```python
from build123d import *

# Parameters (mm, degrees)
F0_R        = 9.525
F1_DEPTH    = 44.45
F2_T1_DEPTH = 44.45
F3_R        = 9.525
F4_W        = 58.7756
F4_H        = 15.875
F5_DEPTH    = 25.4
F6_T1_DEPTH = 12.7


# Not quite as in the source:
# - a fillet or chamfer that OpenCascade refuses, or shapes differently, is made with other operations: its cross-section is extruded or revolved along the edge and cut away or added


with BuildPart() as f1:
    # F0 (on Top) → F1 (new body)
    with BuildSketch(Plane.XY):
        with BuildLine():
            ThreePointArc((0, 19.05), (10.9985226281, 15.5542598667), (17.9605122421, 6.35))
            Line((17.9605122421, 6.35), (88.9, 6.35))
            Line((88.9, 6.35), (88.9, 19.05))
            Line((88.9, 19.05), (0, 19.05))
        make_face()
        with BuildLine():
            ThreePointArc((0, 19.05), (-13.4703841816, -13.4703841816), (19.05, 0))
            ThreePointArc((19.05, 0), (18.7756525614, 3.2213926947), (17.9605122421, 6.35))
            ThreePointArc((17.9605122421, 6.35), (10.9985226281, 15.5542598667), (0, 19.05))
        make_face()
        Circle(F0_R, mode=Mode.SUBTRACT)
    extrude(amount=F1_DEPTH)

    # F2: fillet of radius 6.35 on 1 edges, made by hand

    # F2_s2 → F2_t1 (join)
    with BuildSketch(Plane.XY):
        with BuildLine():
            ThreePointArc((25.4, 6.35), (20.9098719395, 4.4901280605), (19.05, 0))
            ThreePointArc((19.05, 0), (18.7756525614, 3.2213926947), (17.9605122421, 6.35))
            Line((17.9605122421, 6.35), (25.4, 6.35))
        make_face()
    extrude(amount=F2_T1_DEPTH)

    # F3
    f3_edges = [f1.edges().sort_by_distance(p)[0] for p in [
        (88.9, 12.7, 44.45),
        (88.9, 12.7, 0),
    ]]
    fillet(f3_edges, radius=F3_R)

    # F4 (on face) → F5 (cut)
    with BuildSketch(Plane.XZ.offset(-6.35)):
        with Locations((59.5122, 22.2023769543)):
            Rectangle(F4_W, F4_H)
    extrude(amount=-F5_DEPTH, mode=Mode.SUBTRACT)

    # F6: fillet of radius 7.9756 on 2 edges, made by hand

    # F6_s2 → F6_t1 (join)
    with BuildSketch(Plane.XZ.offset(-19.05)):
        with BuildLine():
            ThreePointArc((30.1244, 22.1642769543), (32.460399156, 27.8038777983), (38.1, 30.1398769543))
            Line((38.1, 30.1398769543), (30.1244, 30.1398769543))
            Line((30.1244, 30.1398769543), (30.1244, 22.1642769543))
        make_face()
        with BuildLine():
            ThreePointArc((38.1, 14.2648769543), (32.460399156, 16.6008761102), (30.1244, 22.2404769543))
            Line((30.1244, 22.2404769543), (30.1244, 14.2648769543))
            Line((30.1244, 14.2648769543), (38.1, 14.2648769543))
        make_face()
    extrude(amount=F6_T1_DEPTH)


solid = f1.part
```
For this review, take the finished solid that the model builds, in its own axes (mm). A direction names the side the tool comes from. Coordinates: 2 decimals unless noted, no trailing zeros. Loops run counter-clockwise (first coordinate to the right, second up) from the corner with the lowest first, then second, coordinate; pieces in that order, holes last. Notation, with made-up numbers: (85, 19.25) -> (119, 19.25) arc R17 cw to (119, 29.25) -> close; hole circle Ø11 at (79.5, 66.5). An arc over 180 degrees is marked (long way). Return JSON: item names as keys, results as strings. Group by question number.
(1) Consider section C-C, the plane z = 11.5. Give the boundary of the cut face in (x, y) (3 decimals).
(2) Tool access review of faces 4 (the flat face through (44, 19.05, 32)), 5 (the flat face through (63, 13, 14.265)): name each direction out of +Z, -Z, +X, -X, +Y, -Y from which nothing blocks a thin tool from reaching the whole face with its end or side.
(3) Consider section A-A, the plane x = 56. Give the boundary of the cut face in (y, z).
(4) Consider section B-B, the plane y = -6. Give the boundary of the cut face in (x, z).
(5) For pin 1 Ø1 at (x, z) = (52.5, 14) entering from -Y; pin 2 Ø3 at (y, z) = (-10.5, 32) entering from +X, all flat-tipped, find the tip position at first contact; note any pin that passes through.
(6) To check wall thickness, follow L1, parallel to Y at x = 0, z = 22 (3 decimals); L2, parallel to Z at x = 70, y = 14; L3, parallel to X at y = -0.5, z = 11. State the ranges of each line that lie inside material, in increasing order.
(7) Mouldability with a two-part tool opening along Y and no side actions: class faces 1 (the cylindrical face through (-7.559, -5.796, 21.914)), 2 (the cylindrical face through (32.412, 12.789, 27.755)), 3 (the flat face through (57, 6.35, 32)) as pulls with the +Y half, pulls with the -Y half, needs draft (parallel to the pull), parting line crosses it, or undercut.
Results below:
{
 "1": {"outline": "(0, 19.05) arc R19.05 ccw (long way) to (19.05, 0) arc R6.35 cw to (25.4, 6.35) -> (88.9, 6.35) -> (88.9, 19.05) -> close; hole circle Ø19.05 at (0, 0)"},
 "2": {"face 4": "+Z, -Z, +X, -X, +Y", "face 5": "+X, +Y, -Y"},
 "3": {"outline": "(6.35, 0) -> (19.05, 0) -> (19.05, 14.26) -> (6.35, 14.26) -> close; (6.35, 30.14) -> (19.05, 30.14) -> (19.05, 44.45) -> (6.35, 44.45) -> close"},
 "4": {"outline": "(-18.08, 0) -> (-7.4, 0) -> (-7.4, 44.45) -> (-18.08, 44.45) -> close; (7.4, 0) -> (18.08, 0) -> (18.08, 44.45) -> (7.4, 44.45) -> close"},
 "5": {"pin 1": "stops at y = 6.35", "pin 2": "stops at x = 16.79"},
 "6": {"L1": "y = -19.05 to -9.525, 9.525 to 19.05", "L2": "z = 0 to 14.26, 30.14 to 44.45", "L3": "x = -19.04 to -9.51, 9.51 to 19.04"},
 "7": {"face 1": "undercut", "face 2": "needs draft", "face 3": "pulls with the -Y half"}
}
